Autodesk Inventor part; units mm, degrees
ref_plane "YZ Plane" through (0, 0, 0) normal (1, 0, 0) x (0, 1, 0)
ref_plane "XZ Plane" through (0, 0, 0) normal (0, 1, 0) x (-1, 0, 0)
ref_plane "XY Plane" through (0, 0, 0) normal (0, 0, 1) x (1, 0, 0)
sketch "Эскиз1" plane through (0, 0, 0) normal (0, 1, 0) x (-1, 0, 0)
  line L0 (-77, -87.5) -> (77, -87.5)
  line L1 (90, -74.5) -> (90, 74.5)
  line L2 (77, 87.5) -> (-77, 87.5)
  line L3 (-90, 74.5) -> (-90, -74.5)
  line L4 (90, 0) -> (-90, 0) construction
  line L5 (0, -87.5) -> (0, 87.5) construction
  arc A0 (90, 74.5) -> (77, 87.5) centre (77, 74.5) ccw
  arc A1 (77, -87.5) -> (90, -74.5) centre (77, -74.5) ccw
  arc A2 (-90, -74.5) -> (-77, -87.5) centre (-77, -74.5) ccw
  arc A3 (-77, 87.5) -> (-90, 74.5) centre (-77, 74.5) ccw
  line L6 (75, 83.5) -> (-75, 83.5)
  line L7 (-75, 83.5) -> (-75, 65.5)
  line L8 (-75, 65.5) -> (75, 65.5)
  line L9 (75, 65.5) -> (75, 83.5)
  line L10 (0, 87.5) -> (0, -87.5) construction
  line L11 (75, -83.5) -> (-75, -83.5)
  line L12 (-75, -83.5) -> (-75, -65.5)
  line L13 (-75, -65.5) -> (75, -65.5)
  line L14 (75, -65.5) -> (75, -83.5)
  line L15 (90, 49.8397) -> (90, 20.3597)
  line L16 (0, 65.5) -> (42, 65.5)
  line L17 (90, -32.9125) -> (90, 38.6688)
  line L18 (68, 60) -> (-12, 60)
  line L19 (-12, 60) -> (-12, -60)
  line L20 (-12, -60) -> (68, -60)
  line L21 (68, -60) -> (68, 60)
  line L22 (60, 60) -> (57.2, 60)
  line L23 (60, 57.2) -> (60, 60)
  circle A4 centre (65.2, 57.2) radius 1.5
  line L24 (20, 60) -> (20, -60) construction
  circle A5 centre (65.2, -57.2) radius 1.5
  circle A6 centre (-9.2, 57.2) radius 1.5
  circle A7 centre (-9.2, -57.2) radius 1.5
  line L25 (-20, 0) -> (-25, 0) construction
  line L26 (-25, 0) -> (-81, 0) construction
  line L27 (-13, 42.5) -> (-69, 42.5)
  line L28 (-69, 42.5) -> (-69, -42.5)
  line L29 (-69, -42.5) -> (-13, -42.5)
  line L30 (-13, -42.5) -> (-13, 42.5)
  line L31 (-25, 42.5) -> (-28.7, 42.5)
  line L32 (-25, 38.8) -> (-25, 42.5)
  circle A8 centre (-16.7, 38.8) radius 1.5
  line L33 (-53, 42.5) -> (-53, -42.5) construction
  line L34 (-25, 0) -> (-81, 0) construction
  line L35 (-16.7, 38.8) -> (-16.7, -19.2) construction
  circle A9 centre (-16.7, -19.2) radius 1.5
  circle A10 centre (-65.3, 38.8) radius 1.5
  circle A11 centre (-65.3, -19.2) radius 1.5
  line L36 (90, 60.5) -> (90, 65.5)
  circle A12 centre (65, 60.3847) radius 1.5
  circle A13 centre (65, 52.5) radius 1.5
  line L37 (32.5, 60.3847) -> (32.5, -60) construction
  circle A14 centre (0, 60.3847) radius 1.5
  circle A15 centre (0, 52.5) radius 1.5
  circle A16 centre (-65, 60.3847) radius 1.5
  circle A17 centre (-65, 52.5) radius 1.5
  circle A18 centre (65, -60.3847) radius 1.5
  circle A19 centre (65, -52.5) radius 1.5
  circle A20 centre (0, -60.3847) radius 1.5
  circle A21 centre (0, -52.5) radius 1.5
  circle A22 centre (-65, -60.3847) radius 1.5
  circle A23 centre (-65, -52.5) radius 1.5
  circle A24 centre (86, 0) radius 1.5
  line L38 (86, 0) -> (104.385, 0) construction
  circle A25 centre (72.9998, -13.0002) radius 1.5
  circle A26 centre (72.9998, 12.9998) radius 1.5
  line L39 (90, -19.2) -> (75, -19.2)
  line L40 (75, -19.2) -> (75, 22.1472)
  line L41 (75, 22.1472) -> (90, 22.1472)
  line L42 (90, 22.1472) -> (90, -19.2)
  line L43 (-90, 8.1057) -> (-90, 0)
  line L44 (0, 0) -> (-12, 0)
  line L45 (-12, 5.1924) -> (-12, 5.1924)
  line L46 (75, 78.692) -> (75, 65.5)
  circle A27 centre (81.192, 78.692) radius 1.5
  circle A28 centre (81.192, -78.692) radius 1.5
  circle A29 centre (81.192, 68.692) radius 1.5
  circle A30 centre (81.192, -68.692) radius 1.5
  line L47 (66.2, 9.8) -> (66.2, -10.5)
  line L48 (66.2, -10.5) -> (60.2, -10.5)
  line L49 (60.2, -10.5) -> (60.2, 9.8)
  line L50 (60.2, 9.8) -> (66.2, 9.8)
  circle A31 centre (-81.192, -78.692) radius 1.5
  circle A32 centre (-81.192, 78.692) radius 1.5
  line L51 (0, 0) -> (-71.5, 0) construction
  line L52 (-71.5, 0) -> (-71.5, 45.306) construction
  line L53 (-71.5, 45.306) -> (0, 45.306) construction
  line L54 (0, 45.306) -> (0, 0) construction
  line L55 (-71.5, 45.306) -> (-88, 45.306)
  line L56 (-88, 45.306) -> (-88, 62.3062)
  line L57 (-88, 62.3062) -> (-71.5, 62.3062)
  line L58 (-71.5, 62.3062) -> (-71.5, 45.306)
  line L59 (-71.5, -45.306) -> (-88, -45.306)
  line L60 (-88, -45.306) -> (-88, -62.3062)
  line L61 (-88, -62.3062) -> (-71.5, -62.3062)
  line L62 (-71.5, -62.3062) -> (-71.5, -45.306)
  line L63 (20, -40) -> (-20, -40)
  line L64 (-20, -40) -> (-20, 40)
  line L65 (-20, 40) -> (20, 40)
  line L66 (20, 40) -> (20, -40)
  line L67 (20, 0) -> (-20, 0) construction
  line L68 (0, -40) -> (0, 40) construction
  line L69 (0, 65.5) -> (-4.2, 65.5) construction
  line L70 (-4.2, 65.5) -> (-4.2, 56.5) construction
  line L71 (-4.2, 56.5) -> (0, 56.5) construction
  line L72 (0, 56.5) -> (0, 65.5) construction
  circle A33 centre (-4.2, 56.5) radius 1.5
  line L73 (0, 65.5) -> (-29.4, 65.5) construction
  line L74 (-29.4, 65.5) -> (-29.4, 56.5) construction
  line L75 (-29.4, 56.5) -> (0, 56.5) construction
  line L76 (0, 56.5) -> (0, 65.5) construction
  circle A34 centre (-29.4, 56.5) radius 1.5
  circle A35 centre (-4.2, -56.5) radius 1.5
  circle A36 centre (29.4, -56.5) radius 1.5
  line L77 (0, 60.3847) -> (8.833, 60.3847)
  line L78 (8.833, 60.3847) -> (8.833, 57.162)
  line L79 (8.833, 57.162) -> (0, 57.162)
  line L80 (0, 57.162) -> (0, 60.3847)
  circle A37 centre (8.833, 57.162) radius 1.5
  circle A38 centre (-8.833, 57.162) radius 1.5
  circle A39 centre (8.833, -57.162) radius 1.5
  circle A40 centre (-8.833, -57.162) radius 1.5
  line L81 (-20, 0) -> (-20, -8)
  line L82 (-20, -8) -> (-36, -8)
  line L83 (-36, -8) -> (-36, 8)
  line L84 (-36, 8) -> (-20, 8)
  line L85 (-20, 8) -> (-20, -8)
  line L86 (20, -8) -> (36, -8)
  line L87 (36, -8) -> (36, 8)
  line L88 (36, 8) -> (20, 8)
  line L89 (20, 8) -> (20, -8)
  line L90 (0, 0) -> (16.43, 0) construction
  line L91 (16.43, 0) -> (16.43, 43.8) construction
  line L92 (16.43, 43.8) -> (0, 43.8) construction
  line L93 (0, 43.8) -> (0, 0) construction
  circle A41 centre (16.43, 43.8) radius 1.5
  circle A42 centre (-16.43, 43.8) radius 1.5
  circle A43 centre (16.43, -43.8) radius 1.5
  circle A44 centre (-16.43, -43.8) radius 1.5
  line L94 (0, 0) -> (-32.9, 0) construction
  line L95 (-32.9, 0) -> (-32.9, 46.85) construction
  line L96 (-32.9, 46.85) -> (0, 46.85) construction
  line L97 (0, 46.85) -> (0, 0) construction
  circle A45 centre (-32.9, 46.85) radius 1.5
  point P0 (90, 87.5)
  point P1 (90, -87.5)
  point P2 (-90, 87.5)
  point P3 (-77, -74.5)
  point P4 (60, 0)
  point P5 (75, 0)
  point P6 (60, 0)
  point P7 (-60, 0)
  point P8 (-4, 0)
  point P9 (-5, 0)
  point P10 (-15, 0)
  point P11 (-70, 0)
  point P12 (-14, 0)
  point P13 (-28.7, -19.2)
  point P14 (-17.7, -19.2)
  point P15 (-13, 0)
  point P16 (-14, 0)
  point P17 (-17.6, 40)
  point P18 (-15.8, 40)
  dimension "d0" = 180
  dimension "d1" = 175
  dimension "d2" = 13
  dimension "d7" = 150
  dimension "d8" = 18
  dimension "d13" = 80
  dimension "d14" = 120
  dimension "d21" = 56
  dimension "d22" = 85
  dimension "d25" = 3
  dimension "d26" = 58
  dimension "d27" = 3
  dimension "d30" = 3
  dimension "d32" = 3
  dimension "d33" = 32.5
  dimension "d54" = 3
  dimension "d58" = 3
  dimension "d59" = 3
  dimension "d60" = 15
  dimension "d62" = 12
  dimension "d68" = 3
  dimension "d70" = 3
  dimension "d72" = 20.3
  dimension "d73" = 6
  dimension "d76" = 3
  dimension "d77" = 71.5
  dimension "d78" = 45.306
  dimension "d79" = 40
  dimension "d80" = 80
  dimension "d81" = 4.2
  dimension "d82" = 9
  dimension "d83" = 3
  dimension "d84" = 29.4
  dimension "d85" = 9
  dimension "d86" = 3
  dimension "d87" = 3
  dimension "d88" = 8
  dimension "d89" = 16
  dimension "d90" = 16
  dimension "d91" = 16.43
  dimension "d92" = 43.8
  dimension "d93" = 3
  dimension "d94" = 3
sketch "Эскиз2" plane through (0, 0, 0) normal (0, 1, 0) x (-1, 0, 0)
  line L0 (77, 87.5) -> (-77, 87.5)
  line L1 (-90, 74.5) -> (-90, -74.5)
  line L2 (-77, -87.5) -> (77, -87.5)
  line L3 (90, -74.5) -> (90, 74.5)
  line L4 (90, 0) -> (-90, 0) construction
  line L5 (0, 87.5) -> (0, -87.5) construction
  arc A0 (90, 74.5) -> (77, 87.5) centre (77, 74.5) ccw
  arc A1 (-77, 87.5) -> (-90, 74.5) centre (-77, 74.5) ccw
  arc A2 (-90, -74.5) -> (-77, -87.5) centre (-77, -74.5) ccw
  arc A3 (77, -87.5) -> (90, -74.5) centre (77, -74.5) ccw
  line L6 (150, -150) -> (-150, -150)
  line L7 (-150, -150) -> (-150, 150)
  line L8 (-150, 150) -> (150, 150)
  line L9 (150, 150) -> (150, -150)
  line L10 (150, 0) -> (-150, 0) construction
  line L11 (0, -150) -> (0, 150) construction
  circle A4 centre (0, 0) radius 150
  line L12 (75, -74.5) -> (75, -83.5)
  line L13 (75, -83.5) -> (-75, -83.5)
  line L14 (-75, -83.5) -> (-75, -65.5)
  line L15 (-75, -65.5) -> (75, -65.5)
  line L16 (75, -65.5) -> (75, -83.5)
  line L17 (75, 74.5) -> (75, 83.5)
  line L18 (75, 83.5) -> (-75, 83.5)
  line L19 (-75, 83.5) -> (-75, 65.5)
  line L20 (-75, 65.5) -> (75, 65.5)
  line L21 (75, 65.5) -> (75, 83.5)
  line L22 (0, -65.5) -> (42, -65.5)
  line L23 (42, -65.5) -> (77, -65.5)
  line L24 (77, -65.5) -> (77, -82.3082)
  line L25 (77, -82.3082) -> (42, -82.3082)
  line L26 (77, -65.5) -> (7, -65.5)
  line L27 (7, -65.5) -> (7, -82.3082)
  line L28 (7, -82.3082) -> (77, -82.3082)
  line L29 (77, -82.3082) -> (77, -65.5)
  line L30 (-42, -65.5) -> (-77, -65.5)
  line L31 (-77, -65.5) -> (-77, -82.3082)
  line L32 (-7, -65.5) -> (-7, -82.3082)
  line L33 (-7, -82.3082) -> (-77, -82.3082)
  line L34 (42, -65.5) -> (29.5, -65.5)
  line L35 (29.5, -10.5) -> (54.5, -10.5)
  line L36 (54.5, -10.5) -> (54.5, -65.5)
  line L37 (54.5, -65.5) -> (29.5, -65.5)
  line L38 (29.5, -65.5) -> (29.5, -10.5)
  line L39 (29.5, 10.5) -> (54.5, 10.5)
  line L40 (54.5, 10.5) -> (54.5, 65.5)
  line L41 (29.5, 65.5) -> (29.5, 10.5)
  line L42 (-29.5, -10.5) -> (-54.5, -10.5)
  line L43 (-54.5, -10.5) -> (-54.5, -65.5)
  line L44 (-29.5, -65.5) -> (-29.5, -10.5)
  line L45 (-29.5, 65.5) -> (-29.5, 10.5)
  line L46 (-29.5, 10.5) -> (-54.5, 10.5)
  line L47 (-54.5, 10.5) -> (-54.5, 65.5)
  point P0 (0, 0)
  point P1 (-90, -87.5)
  point P2 (-90, 87.5)
  point P3 (90, -87.5)
  point P4 (-80.411, -84.4848)
  point P5 (77, 74.5)
  point P6 (-7, -73.9041)
  point P7 (7, -73.9041)
  dimension "d34" = 180
  dimension "d35" = 175
  dimension "d36" = 13
  dimension "d37" = 300
  dimension "d38" = 300
  dimension "d41" = 150
  dimension "d42" = 18
  dimension "d44" = 35
  dimension "d45" = 70
  dimension "d46" = 14
  dimension "d47" = 84
  dimension "d50" = 25
extrude "Выдавливание1" add sketch "Эскиз1" along normal blind 2 contours A2 L3 A3 L2 A0 L1 L41 L40 L39 A1 L0 | L39 L40 L41 L1 | L18 A12 L21 L20 A18 A20 L19 L63 L66 L86 L87 L88 L65 A14 L80 L79 A37 L78 | L78 A37 L79 L80 A14 L18 | L18 A14 L77 L78 | L65 A8 L64 L84 L83 L82 L63 L30 L29 A44 L28 L27 A42 | L65 A8 | A4 | A5 | A38 A6 | A40 A7 | A10 | A11 picked at (-16.908, 40.0547) picked at (-10.5675, 57.2211) picked at (-10.5675, -57.2211)
chamfer "Фаска1" distance 1.5 angle 45 3 edges at (-84.5, 2, 0) (-71.4998, 2, -13.0002) (-71.4998, 2, 12.9998)
chamfer "Фаска2" distance 1.5 angle 45 23 edges at (-79.692, 0, 78.692) (-79.692, 0, 68.692) (-79.692, 0, -78.692) (-79.692, 0, -68.692) (-63.5, 2, 60.3847) (-63.5, 2, 52.5) (1.5, 2, 60.3847) (1.5, 2, 52.5) (66.5, 2, 52.5) (66.5, 2, 60.3847) (66.5, 2, -60.3847) (66.5, 2, -52.5) (1.5, 2, -52.5) (1.5, 2, -60.3847) (-63.5, 2, -60.3847) (-63.5, 2, -52.5) (-7.333, 0, -57.162) (10.333, 0, -57.162) (-7.333, 0, 57.162) (10.333, 0, 57.162) (82.692, 0, 78.692) (82.692, 0, -78.692) (34.4, 0, 46.85)
properties part number "base_ls"
Could you check a few things on this model? Use its own coordinates, in mm. Give positions to 0.01 mm unless a question says otherwise; leave off trailing zeros. Return JSON: item names as keys, results as strings. Group by question number.
Q1. Please list where these lines run through material, in increasing order: line 1 along Z through (x, y) = (-43, 0.3); line 2 along X through (y, z) = (0.8, -5); line 3 along Z through (x, y) = (-18.5, 0.4). Write a range as [from, to].
Q2. Thinking about a two-plate mould opening in Z: for faces 1 (the face through (-71, 1, -13)), 2 (the face through (21, 2, -18)), which applies, pulls with the +Z half, pulls with the -Z half, needs draft (parallel to the pull), parting line crosses it, or undercut?
Q3. Will these pins go through, and if not, where does the flat tip stop? pin 1 Ø2.5 at (x, z) = (-65, -60.38) entering from +Y; pin 2 Ø4 at (x, z) = (-81.192, 78.692) entering from -Y; pin 3 Ø3.5 at (x, z) = (81.192, 78.692) entering from -Y.
Q4. Suppose I cut it at A-A, the plane y = 0.95. State how many separate pieces and enclosed holes the cut face has, and give its area (3 significant figures).
Resolved:
{
 "1": {"line 1": "z = [-87.5, -83.5], [-65.5, 65.5], [83.5, 87.5]", "line 2": "x = [-90, -66.2], [-60.2, -36], [36, 90]", "line 3": "z = [-87.5, -83.5], [-65.5, -40], [40, 65.5], [83.5, 87.5]"},
 "2": {"face 1": "undercut", "face 2": "needs draft"},
 "3": {"pin 1": "passes through", "pin 2": "stops at y = 1", "pin 3": "stops at y = 1.25"},
 "4": {"separate pieces": "1", "enclosed holes": "40", "area": "21,200 mm2"}
}
